CAD build for the part. Positions are in the model's coordinates, mm. A direction names the side the tool comes from. Round coordinates to 2 decimals unless told otherwise and drop trailing zeros. Order: outer loops, then holes, each group sorted by start corner. A loop starts at its lowest first (then second) coordinate and runs counter-clockwise, first axis right, second up. Notation, with made-up numbers: (-8.75, -39) -> (31.25, -39) arc R13 cw to (31.25, -17) -> close; hole circle Ø4 at (-27, -19). An arc over 180 degrees is marked (long way). Return JSON: item names as keys, results as strings. Group by question number.
Q1. Cut at D-D (x = -1.5). Write the cut outline in (y, z) (3 decimals).
Q2. Cut at B-B (y = -12.7). Write the cut outline in (x, z), then the cut area to 3 significant figures.
Q3. Cut at A-A (x = 3.77). Write the cut outline in (y, z) (3 decimals).
Q4. Which spindle directions (+Z, -Z, +X, -X, +Y, -Y) get a long thin tool onto all of the face, cutting with end or side? Do faces 4 (the flat face through (0, 0, 2)), 5 (the flat face through (8.97, 0, 1)), 6 (the flat face through (0, -16.335, -4)). Say none if no direction does.
Q5. Probe line 1 along Y through (x, z) = (3.77, 1.45) (3 decimals); line 2 along Y through (x, z) = (3.77, -0.5) (3 decimals); line 3 along Y through (x, z) = (-8, -0.25) (3 decimals). List the from-to ranges inside material, lowest first.
Q6. Mould opens along Y. For faces 1 (the flat face through (0, 18.735, -3)), 2 (the flat face through (11, 12.535, 1)), 3 (the flat face through (-16, 0, -8)) say: +Y half, -Y half, draft (parallel to the pull), parting line (faces both ways), or undercut.
Q7. Flat gauge pin, fed straight in: pin 1 (4 mm diameter, centred on x = 3.77, y = -12.7, fed in from -Z). Where does the tip first touch, or does it go through?
Q8. Cut at C-C (z = 0.75). Write the cut outline in (x, y) (3 decimals).
from build123d import *

# Parameters (mm, degrees)
F0_W     = 34.86
F0_H     = 37.47
F0_R     = 2.8
F0_W_2   = 4.5
F0_H_2   = 6.7
F0_R_2   = 1.6
F1_DEPTH = 2
F2_DEPTH = 8
F3_DEPTH = 2


with BuildPart() as f1:
    # F0 (on Top) → F1 (new body)
    with BuildSketch(Plane.XY):
        Rectangle(F0_W, F0_H)
        Polygon((15.03, 16.335), (15.03, -16.335), (-15.03, -16.335), (-15.03, -14.065), (-15.03, 3.565), (-15.03, 16.335), align=None, mode=Mode.SUBTRACT)
        Polygon((-15.03, -16.335), (15.03, -16.335), (15.03, 16.335), (-15.03, 16.335), (-15.03, 3.565), (-8.03, 3.565), (-8.03, -5.735), (-10.53, -5.735), (-10.53, -14.065), (-14.03, -14.065), (-15.03, -14.065), align=None)
        with Locations((3.77, -12.7)):
            Circle(F0_R, mode=Mode.SUBTRACT)
        with Locations((11.22, -8.785)):
            Rectangle(F0_W_2, F0_H_2, mode=Mode.SUBTRACT)
        with Locations((11.22, 0.235)):
            Rectangle(F0_W_2, F0_H_2, mode=Mode.SUBTRACT)
        with Locations((11.22, 9.185)):
            Rectangle(F0_W_2, F0_H_2, mode=Mode.SUBTRACT)
        with Locations((3.77, 12.7)):
            Circle(F0_R, mode=Mode.SUBTRACT)
        with Locations((3.77, 12.7)):
            Circle(F0_R)
        with Locations((3.77, 12.7)):
            Circle(F0_R_2, mode=Mode.SUBTRACT)
        with Locations((3.77, -12.7)):
            Circle(F0_R)
        with Locations((3.77, -12.7)):
            Circle(F0_R_2, mode=Mode.SUBTRACT)
    extrude(amount=F1_DEPTH)

    # F0 (on Top) → F2 (join)
    with BuildSketch(Plane.XY):
        Rectangle(F0_W, F0_H)
        Polygon((15.03, 16.335), (15.03, -16.335), (-15.03, -16.335), (-15.03, -14.065), (-15.03, 3.565), (-15.03, 16.335), align=None, mode=Mode.SUBTRACT)
    extrude(amount=-F2_DEPTH)

    # F0 (on Top) → F3 (join)
    with BuildSketch(Plane.XY):
        with Locations((3.77, 12.7)):
            Circle(F0_R)
        with Locations((3.77, 12.7)):
            Circle(F0_R_2, mode=Mode.SUBTRACT)
        with Locations((3.77, -12.7)):
            Circle(F0_R)
        with Locations((3.77, -12.7)):
            Circle(F0_R_2, mode=Mode.SUBTRACT)
    extrude(amount=-F3_DEPTH)


solid = f1.part
Solution:
{
 "1": {"outline": "(-18.735, -8) -> (-16.335, -8) -> (-16.335, 0) -> (16.335, 0) -> (16.335, -8) -> (18.735, -8) -> (18.735, 2) -> (-18.735, 2) -> close"},
 "2": {"outline": "(-17.43, -8) -> (-15.03, -8) -> (-15.03, 2) -> (-17.43, 2) -> close; (-10.53, 0) -> (0.97, 0) -> (0.97, -2) -> (2.17, -2) -> (2.17, 2) -> (-10.53, 2) -> close; (5.37, -2) -> (6.57, -2) -> (6.57, 0) -> (15.03, 0) -> (15.03, -8) -> (17.43, -8) -> (17.43, 2) -> (5.37, 2) -> close", "area": "97.5 mm²"},
 "3": {"outline": "(-18.735, -8) -> (-16.335, -8) -> (-16.335, 0) -> (-15.5, 0) -> (-15.5, -2) -> (-14.3, -2) -> (-14.3, 2) -> (-18.735, 2) -> close; (-11.1, -2) -> (-9.9, -2) -> (-9.9, 0) -> (9.9, 0) -> (9.9, -2) -> (11.1, -2) -> (11.1, 2) -> (-11.1, 2) -> close; (14.3, -2) -> (15.5, -2) -> (15.5, 0) -> (16.335, 0) -> (16.335, -8) -> (18.735, -8) -> (18.735, 2) -> (14.3, 2) -> close"},
 "4": {"face 4": "+Z, +X, -X, +Y, -Y", "face 5": "+Z, -Z", "face 6": "-Z"},
 "5": {"line 1": "y = -18.735 to -14.3, -11.1 to 11.1, 14.3 to 18.735", "line 2": "y = -18.735 to -16.335, -15.5 to -14.3, -11.1 to -9.9, 9.9 to 11.1, 14.3 to 15.5, 16.335 to 18.735", "line 3": "y = -18.735 to -16.335, 16.335 to 18.735"},
 "6": {"face 1": "+Y half", "face 2": "undercut", "face 3": "draft"},
 "7": {"pin 1": "stops at z = -2"},
 "8": {"outline": "(-17.43, -18.735) -> (17.43, -18.735) -> (17.43, 18.735) -> (-17.43, 18.735) -> close; hole (-15.03, -14.065) -> (-10.53, -14.065) -> (-10.53, -5.735) -> (-8.03, -5.735) -> (-8.03, 3.565) -> (-15.03, 3.565) -> close; hole circle Ø3.2 at (3.77, -12.7); hole circle Ø3.2 at (3.77, 12.7); hole (8.97, -12.135) -> (13.47, -12.135) -> (13.47, -5.435) -> (8.97, -5.435) -> close; hole (8.97, -3.115) -> (13.47, -3.115) -> (13.47, 3.585) -> (8.97, 3.585) -> close; hole (8.97, 5.835) -> (13.47, 5.835) -> (13.47, 12.535) -> (8.97, 12.535) -> close"}
}
